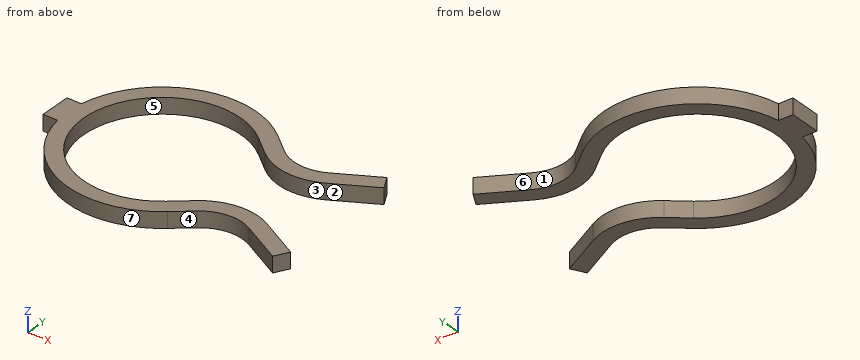
from build123d import *

# Parameters (mm, degrees)
EXTRUDE1_DEPTH = 5.08


with BuildPart() as part:
    # Sketch1 → Extrude1 (new body)
    with BuildSketch(Plane.XY):
        with BuildLine():
            Line((16.277171033, 19.499069289), (22.162906601, 14.585854045))
            ThreePointArc((22.162906601, 14.585854045), (32.529038116, 10.249394717), (43.535952824, 12.509790851))
            Line((43.535952824, 12.509790851), (56.757436861, 19.765747267))
            Line((56.757436861, 19.765747267), (54.313392075, 24.219177976))
            Line((54.313392075, 24.219177976), (41.091908038, 16.963221561))
            ThreePointArc((41.091908038, 16.963221561), (33.020170585, 15.305597729), (25.418340808, 18.485667902))
            Line((25.418340808, 18.485667902), (19.53260524, 23.398883147))
            ThreePointArc((19.53260524, 23.398883147), (-10.562606276, 28.591287985), (-30.053685298, 5.08))
            Line((-30.053685298, 5.08), (-34.776815298, 5.08))
            Line((-34.776815298, 5.08), (-34.776815298, -5.08))
            Line((-34.776815298, -5.08), (-30.053685298, -5.08))
            ThreePointArc((-30.053685298, -5.08), (-10.562606276, -28.591287985), (19.53260524, -23.398883147))
            Line((19.53260524, -23.398883147), (25.418340808, -18.485667902))
            ThreePointArc((25.418340808, -18.485667902), (33.020170585, -15.305597729), (41.091908038, -16.963221561))
            Line((41.091908038, -16.963221561), (54.313392075, -24.219177976))
            Line((54.313392075, -24.219177976), (56.757436861, -19.765747267))
            Line((56.757436861, -19.765747267), (43.535952824, -12.509790851))
            ThreePointArc((43.535952824, -12.509790851), (32.529038116, -10.249394717), (22.162906601, -14.585854045))
            Line((22.162906601, -14.585854045), (16.277171033, -19.499069289))
            ThreePointArc((16.277171033, -19.499069289), (-25.4, 0), (16.277171033, 19.499069289))
        make_face()
    extrude(amount=EXTRUDE1_DEPTH)


solid = part.part
Model file for the job. Use its own axes, mm. Face numbers are marked on the shaded views. A direction names the side the tool comes from. Give positions to 0.01 mm unless a question says otherwise; leave off trailing zeros. Order: outer loops, then holes, each group sorted by start corner. A loop starts at its lowest first (then second) coordinate and runs counter-clockwise, first axis right, second up. Notation, with made-up numbers: (39.25, -14.75) - (46.25, -14.75) arc R23 ccw to (46.25, 8.25) - close; hole circle Ø1 at (-12, -16.75). An arc over 180 degrees is marked (long way). Write item = value, one per line. Start each with the question number.
1. Two-plate mould, pull along Y, no slides. Class the marked faces 5, 6 and 7: pulls with the +Y half, pulls with the -Y half, needs draft (parallel to the pull), parting line crosses it, or undercut.
2. Cut at B-B, the plane z = 3.5. List the corners of the cut face in (x, y).
3. Probe line 1 along Y through (x, z) = (0, 1.4); line 2 along X through (y, z) = (-18.5, 1.85); line 3 along X through (y, z) = (16.5, 4.65). List the from-to ranges inside material, lowest first.
4. Cut at D-D, the plane y = 0. List the corners of the cut face in (x, z), and give its area (3 significant figures).
5. Cut at C-C, the plane x = 27. List the corners of the cut face in (y, z).
6. Drop flat-ended pins along their axis: P1, Ø1, axis at x = 45.5, z = 3, coming from the +Y side; P2, Ø1, axis at y = 9.5, z = 4.5, coming from the +X side; P3, Ø1.5, axis at y = 16, z = 2.5, coming from the +X side. Give the stop position or say it passes through.
7. Which spindle directions (+Z, -Z, +X, -X, +Y, -Y) get a long thin tool onto all of the face, cutting with end or side? Do the marked faces 1, 2, 3 and 4. Say none if no direction does.
8. Cut at A-A, the plane x = 0. List the corners of the cut face in (y, z).
Taken from the geometry:
q1.face_5 = undercut
q1.face_6 = pulls with the +Y half
q1.face_7 = pulls with the -Y half
q2.outline = (-34.78, -5.08) - (-30.05, -5.08) arc R30.48 ccw to (19.53, -23.4) - (25.42, -18.49) arc R13.97 cw to (41.09, -16.96) - (54.31, -24.22) - (56.76, -19.77) - (43.54, -12.51) arc R19.05 ccw to (22.16, -14.59) - (16.28, -19.5) arc R25.4 cw (long way) to (16.28, 19.5) - (22.16, 14.59) arc R19.05 ccw to (43.54, 12.51) - (56.76, 19.77) - (54.31, 24.22) - (41.09, 16.96) arc R13.97 cw to (25.42, 18.49) - (19.53, 23.4) arc R30.48 ccw to (-30.05, 5.08) - (-34.78, 5.08) - close
q3.line_1 = -30.48 to -25.4, 25.4 to 30.48
q3.line_2 = -24.22 to -17.4, 17.47 to 25.4, 43.89 to 54.45
q3.line_3 = -25.63 to -19.31, 19.87 to 28.57, 40.17 to 50.81
q4.outline = (-34.78, 0) - (-25.4, 0) - (-25.4, 5.08) - (-34.78, 5.08) - close
q4.area = 47.6 mm²
q5.outline = (-17.34, 0) - (-11.64, 0) - (-11.64, 5.08) - (-17.34, 5.08) - close; (11.64, 0) - (17.34, 0) - (17.34, 5.08) - (11.64, 5.08) - close
q6.P1 = 19.66
q6.P2 = -23.35
q6.P3 = 51.26
q7.face_1 = +Z, -Z, +Y
q7.face_2 = +Z, -Z, +X
q7.face_3 = +Z, -Z
q7.face_4 = +Z, -Z, -Y
q8.outline = (-30.48, 0) - (-25.4, 0) - (-25.4, 5.08) - (-30.48, 5.08) - close; (25.4, 0) - (30.48, 0) - (30.48, 5.08) - (25.4, 5.08) - close
